Autodesk Inventor part; units mm, degrees
ref_plane "YZ Plane" through (0, 0, 0) normal (1, 0, 0) x (0, 1, 0)
ref_plane "XZ Plane" through (0, 0, 0) normal (0, 1, 0) x (-1, 0, 0)
ref_plane "XY Plane" through (0, 0, 0) normal (0, 0, 1) x (1, 0, 0)
sketch "Sketch1" plane through (0, 0, 0) normal (0, 0, 1) x (1, 0, 0)
  line L0 (-6.35, 3.6662) -> (0, 7.3323)
  line L1 (0, 7.3323) -> (6.35, 3.6662)
  line L2 (6.35, 3.6662) -> (6.35, -3.6662)
  line L3 (6.35, -3.6662) -> (0, -7.3323)
  line L4 (0, -7.3323) -> (-6.35, -3.6662)
  line L5 (-6.35, -3.6662) -> (-6.35, 3.6662)
  arc A0 (9.525, 0.0229) -> (-9.5205, 0.2942) centre (0, 0) ccw
  arc A1 (-38.1, -50.8) -> (-9.5205, 0.2942) centre (-72.9901, 2.2559) ccw
  arc A2 (-38.1, -50.8) -> (9.525, 0.0229) centre (-41.2749, -0.0993) ccw
  dimension "d0" = 12.7
  dimension "d1" = 38.1
  dimension "d2" = 19.05
  dimension "d3" = 50.8
  dimension "d4" = 63.5
  dimension "d5" = 50.8
extrude "Extrusion1" add sketch "Sketch1" along normal mid plane 152.4
fillet "Fillet1" radius 3.175 1 edges at (-38.1, -50.8, 0)
properties part number "PLATE,TEARDROP,DROPBAR" material "ABS Plastic"
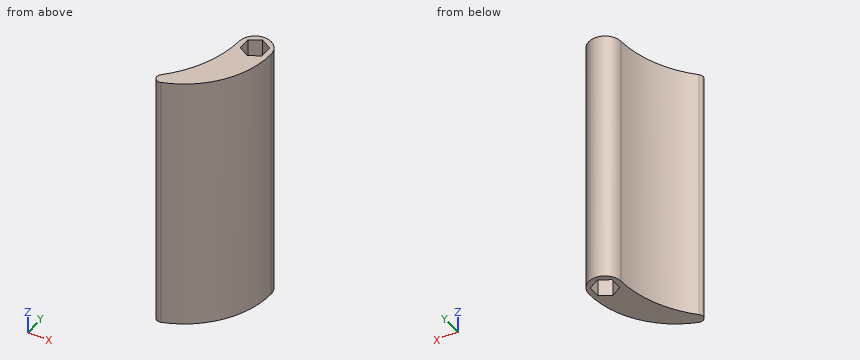
Work out the finished part from the listing and answer in its coordinate system (mm). Coordinates: 2 decimals unless noted, no trailing zeros. Write each loop counter-clockwise with the first axis right and the second up, starting at its lowest first coordinate (ties: lowest second). Pieces come first, ordered by that corner, then holes. Notation, with made-up numbers: M 44,29.25 L 94,29.25 A13 cw 94,35.25 Z; hole C 38,80 d1. An arc over 180 degrees is marked long. Answer as CSV lines item,"result". Start each with the question number.
Item 1: Consider L1, parallel to X at y = 0, z = 53.5; L2, parallel to Y at x = -1, z = 54.5; L3, parallel to Y at x = 4, z = 40.5. Determine where each line is inside the solid, lowest interval first.
Item 2: Section B-B on x = -23 is taken. Write down the section's boundary in (y, z), and give its area (3 significant figures).
Item 3: Section A-A on x = -3.5 is taken. Write down the section's boundary in (y, z), and give its area (3 significant figures).
Item 4: Flat-ended cylindrical pins translate along their axes: P1, Ø8, axis at x = 1.5, z = 1, coming from the -Y side; P2, Ø1, axis at y = -12.5, z = 47.5, coming from the -X side; P3, Ø3, axis at y = -12, z = -31.5, coming from the -X side; P4, Ø6, axis at x = -14, y = -0.5, coming from the -Z side. Find the tip coordinate at first contact, or state that the pin passes through.
Item 5: Section C-C on y = -16.5 is taken. Write down the section's boundary in (x, z).
Checks:
1,L1,"x = -9.53 to -6.35, 6.35 to 9.53"
1,L2,"y = -31.06 to -6.75, 6.75 to 9.47"
1,L3,"y = -23.14 to -5.02, 5.02 to 8.64"
2,outline,"M -47.5,-76.2 L -36.9,-76.2 L -36.9,76.2 L -47.5,76.2 Z"
2,area,"1,620 mm²"
3,outline,"M -34.07,-76.2 L -5.31,-76.2 L -5.31,76.2 L -34.07,76.2 Z; M 5.31,-76.2 L 8.86,-76.2 L 8.86,76.2 L 5.31,76.2 Z"
3,area,"4,920 mm²"
4,P1,"stops at y = -32.92"
4,P2,"stops at x = -11.35"
4,P3,"stops at x = -11.48"
4,P4,"passes through"
5,outline,"M -12.32,-76.2 L 6.8,-76.2 L 6.8,76.2 L -12.32,76.2 Z"
